```python
from build123d import *

# Parameters (mm, degrees)
F2_SIZE = 2
F3_SIZE = 1


with BuildPart() as f1:
    # F0 (on Front) → F1 (revolve)
    with BuildSketch(Plane.XZ):
        Polygon((0, 13.5), (0, 4), (20, 4), (20, 20.5), (-50, 20.5), (-50, 13.5), (-3, 13.5), (-3, 16.5), (0, 16.5), align=None)
    revolve(axis=Axis((-15.148313, 0, 0), (-1, 0, 0)))

    # F2
    f2_edges = [f1.edges().sort_by_distance(p)[0] for p in [
        (-50, 0, -20.5),
        (20, 0, -20.5),
    ]]
    chamfer(f2_edges, length=F2_SIZE)

    # F3
    f3_edges = [f1.edges().sort_by_distance(p)[0] for p in [
        (-50, 0, -13.5),
        (20, 0, -4),
    ]]
    chamfer(f3_edges, length=F3_SIZE)


solid = f1.part
```
For this review, take the finished solid that the model builds, in its own axes (mm). A direction names the side the tool comes from. Give positions to 0.01 mm unless a question says otherwise; leave off trailing zeros. Write each loop counter-clockwise with the first axis right and the second up, starting at its lowest first coordinate (ties: lowest second). Pieces come first, ordered by that corner, then holes. Notation, with made-up numbers: M 28,45.5 L 42,45.5 A32 ccw 42,79.5 Z; hole C -10.5,41.5 d5. An arc over 180 degrees is marked long. Answer as a JSON object with one key per item and string values. Group by question number.
Item 1: Draft analysis for pull direction X (two halves, no side actions). For faces 4 (the flat face through (-3, 0, 14)), 5 (the flat face through (20, -4, -4)), 6 (the cylindrical face through (9.633, -3.905, -0.867)), 7 (the cylindrical face through (-1.48, -6.32, 15.24)), state which applies: +X half, -X half, draft (parallel to the pull), parting line (faces both ways), or undercut.
Item 2: For pin 1 Ø4 at (x, y) = (-4, 11) entering from +Z; pin 2 Ø10 at (x, z) = (-34.5, -2.5) entering from +Y; pin 3 Ø12 at (x, y) = (-41.5, 10.5) entering from -Z, all flat-tipped, find the tip position at first contact; note any pin that passes through.
Item 3: Tool access review of faces 1 (the cylindrical face through (-25.68, -13.18, -2.93)), 2 (the cylindrical face through (-15.462, -20.013, -4.444)), 3 (the flat face through (0, -3, 3)): name each direction out of +Z, -Z, +X, -X, +Y, -Y from which nothing blocks a thin tool from reaching the whole face with its end or side.
Item 4: Consider section A-A on y = 0. Write out the cut boundary in (x, z), plus the area to 3 significant figures.
Item 5: For probe 1 along X at (y, z) = (13.5, 6); probe 2 along Y at (x, z) = (-0.7, 0); probe 3 along Y at (x, z) = (-26, 0), list the stretches that pass through material, from the lowest coordinate up. Write a range as [from, to].
Item 6: Consider section C-C on x = -37. Write out the cut boundary in (y, z).
Check result:
{
 "1": {"face 4": "undercut", "face 5": "+X half", "face 6": "draft", "face 7": "undercut"},
 "2": {"pin 1": "stops at z = 18.42", "pin 2": "stops at y = 20.5", "pin 3": "stops at z = -20"},
 "3": {"face 1": "-X", "face 2": "+X, -X", "face 3": "none"},
 "4": {"outline": "M -50,-18.5 L -48,-20.5 L 18,-20.5 L 20,-18.5 L 20,-5 L 19,-4 L 0,-4 L 0,-16.5 L -3,-16.5 L -3,-13.5 L -49,-13.5 L -50,-14.5 Z; M -50,14.5 L -49,13.5 L -3,13.5 L -3,16.5 L 0,16.5 L 0,4 L 19,4 L 20,5 L 20,18.5 L 18,20.5 L -48,20.5 L -50,18.5 Z", "area": "1,330 mm^2"},
 "5": {"probe 1": "x = [-50, -3], [0, 20]", "probe 2": "y = [-20.5, -16.5], [16.5, 20.5]", "probe 3": "y = [-20.5, -13.5], [13.5, 20.5]"},
 "6": {"outline": "C 0,0 d41; hole C 0,0 d27"}
}
